```python
from build123d import *

# Parameters (mm, degrees)
SKETCH013_R     = 2.568486
PAD009_DEPTH    = 2.7
PAD009_FACE24_R = 2.568486
PAD010_DEPTH    = 6
SKETCH014_W     = 26.409815
SKETCH014_H     = 3.3
POCKET002_DEPTH = 17.5
FILLET004_R     = 15
FILLET005_R     = 4
FILLET006_R     = 6


with BuildPart() as part:
    # Sketch013 → Pad009 (new body)
    with BuildSketch(Plane.YZ.offset(2.7)):
        Polygon((20.516043, -0.037444), (30.366142, -1.649044), (35.213383, -1.649044), (36.83709, -1.959458), (38.007114, -2.29375), (38.389164, -2.413141), (39.177135, -2.866822), (39.72633, -3.224993), (40.275524, -3.63092), (40.967991, -4.299505), (41.254524, -4.729309), (41.923111, -5.636675), (41.923111, -12.869325), (41.062038, -14.015471), (40.035282, -14.922836), (39.032402, -15.710812), (37.838501, -16.236128), (36.525211, -16.133759), (35.140285, -16.133759), (6.593163, -16.133759), (-3.283293, -7.56256), (-3.283293, -0.110564), align=None)
        with Locations((35.551899, -9.23625)):
            Circle(SKETCH013_R, mode=Mode.SUBTRACT)
    extrude(amount=-PAD009_DEPTH)

    # Pad009 Face24 → Pad010 (add)
    with BuildSketch(Plane(origin=(2.7, 19.058053, -8.03373), x_dir=(0, -1, 0), z_dir=(1, 0, 0))):
        Polygon((-11.308089, -6.384686), (-1.45799, -7.996286), (22.341346, -7.923166), (22.341346, -0.47117), (12.46489, 8.100029), (-16.082232, 8.100029), (-17.467158, 8.100029), (-18.780448, 8.202398), (-19.974349, 7.677082), (-20.977229, 6.889106), (-22.003985, 5.981741), (-22.865058, 4.835595), (-22.865058, -2.397055), (-22.196471, -3.304421), (-21.909938, -3.734225), (-21.217471, -4.40281), (-20.668277, -4.808737), (-20.119082, -5.166908), (-19.331111, -5.620589), (-18.949061, -5.73998), (-17.779037, -6.074272), (-16.15533, -6.384686), align=None)
        with Locations((-16.493846, 1.20252)):
            Circle(PAD009_FACE24_R, mode=Mode.SUBTRACT)
    extrude(amount=PAD010_DEPTH)

    # Sketch014 (on Face46 of Pad010) → Pocket002 (cut, symmetric)
    with BuildSketch(Plane.YX.offset(16.133759)):
        with Locations((33.765693, 4.35)):
            Rectangle(SKETCH014_W, SKETCH014_H)
    extrude(amount=POCKET002_DEPTH, both=True, mode=Mode.SUBTRACT)

    # Fillet004
    fillet004_edges = [part.edges().sort_by_distance(p)[0] for p in [
        (5.7, 6.593163, -16.133759),
    ]]
    fillet(fillet004_edges, radius=FILLET004_R)

    # Fillet005
    fillet005_edges = [part.edges().sort_by_distance(p)[0] for p in [
        (4.35, 20.560785, -16.133759),
    ]]
    fillet(fillet005_edges, radius=FILLET005_R)

    # Fillet006
    fillet006_edges = [part.edges().sort_by_distance(p)[0] for p in [
        (5.7, -3.283293, -7.56256),
    ]]
    fillet(fillet006_edges, radius=FILLET006_R)


with BuildPart() as part_1:
    # Body005 placement: moved
    add(part.part.moved(Location((26.9, 0, 0))))


solid = part_1.part
```
For this review, take the finished solid that the model builds, in its own axes (mm). A direction names the side the tool comes from. Round coordinates to 2 decimals unless told otherwise and drop trailing zeros. Write each loop counter-clockwise with the first axis right and the second up, starting at its lowest first coordinate (ties: lowest second). Pieces come first, ordered by that corner, then holes. Notation, with made-up numbers: (61.25, 48) -> (68.25, 48) arc R12 ccw to (68.25, 69) -> close; hole circle Ø10 at (1.5, 59). An arc over 180 degrees is marked (long way). Use one line per item in the form item = value.
Q1. Consider section C-C (x = 31.75). State the section outline as (y, z) points.
Resolved:
outline = (-3.28, -4.83) arc R6 ccw to (-1.22, -9.36) -> (2.36, -12.46) arc R15 ccw to (12.19, -16.13) -> (16.56, -16.13) arc R4 ccw to (20.56, -12.13) -> (20.56, -0.04) -> (20.52, -0.04) -> (-3.28, -0.11) -> close
Q2. To check wall thickness, follow probe 1 along X at (y, z) = (24, -3.25); probe 2 along Y at (x, z) = (30.5, -4.75); probe 3 along Y at (x, z) = (28.25, -7). State the ranges of each line that lie inside material, in increasing order. Write a range as from..to.
Resolved:
probe_1 = 26.9..29.6, 32.9..35.6
probe_2 = -3.28..20.56
probe_3 = -2.88..34.29, 36.82..41.92
Q3. The part is to be moulded in two halves that separate along Y. For faces 6 (the cylindrical face through (31.311, 7.017, -15.212)), 7 (the flat face through (34.2, 36, -1.8)), 8 (the cylindrical face through (28.269, 36.737, -11.515)), say which applies: released by +Y, released by -Y, zero draft, split by the parting line, or undercut.
Resolved:
face_6 = released by -Y
face_7 = released by +Y
face_8 = undercut
Q4. Machinability: for faces 1 (the flat face through (31, -3.283, -2)), 2 (the flat face through (28, 33, -1.649)), 3 (the flat face through (28.231, 40.541, -14.476)), 4 (the flat face through (29, 24, -16.134)), 5 (the flat face through (31, 20.561, -6)), which of the approach directions +Z, -Z, +X, -X, +Y, -Y give a long, thin tool a straight path to every point of the face, cutting with its end or side? Answer none if there is none.
Resolved:
face_1 = +Z, -Z, +X, -X, -Y
face_2 = +Z, +X, -X, +Y
face_3 = -Z, +X, -X, +Y
face_4 = -Z, +X, -X, -Y
face_5 = +Z, -Z, +Y
Q5. Consider section D-D (x = 34.25). State the section outline as (y, z) points (1 decimal).
Resolved:
outline = (-3.3, -4.8) arc R6 ccw to (-1.2, -9.4) -> (2.4, -12.5) arc R15 ccw to (12.2, -16.1) -> (36.5, -16.1) -> (37.8, -16.2) -> (39, -15.7) -> (40, -14.9) -> (41.1, -14) -> (41.9, -12.9) -> (41.9, -5.6) -> (41.3, -4.7) -> (41, -4.3) -> (40.3, -3.6) -> (39.7, -3.2) -> (39.2, -2.9) -> (38.4, -2.4) -> (38, -2.3) -> (36.8, -2) -> (35.2, -1.6) -> (30.4, -1.6) -> (20.5, 0) -> (-3.3, -0.1) -> close; hole circle Ø5.1 at (35.6, -9.2)
Q6. Clearance check with flat-ended pins moving along their axes: pin 1 Ø1.4 at (x, y) = (35, 32.5) entering from +Z; pin 2 Ø3 at (y, z) = (35.55, -9.24) entering from -X; pin 3 Ø4 at (x, y) = (31.5, 32.5) entering from -Z. State where each tip first meets the part, or that it passes through.
Resolved:
pin_1 = -1.65
pin_2 = through
pin_3 = -16.13
Q7. Consider section B-B (z = -10). State the section outline as (x, y) points.
Resolved:
outline = (26.9, -0.47) -> (35.6, -0.47) -> (35.6, 33.1) -> (32.9, 33.1) -> (32.9, 20.56) -> (29.6, 20.56) -> (29.6, 33.1) -> (26.9, 33.1) -> close; (26.9, 38) -> (29.6, 38) -> (29.6, 41.92) -> (26.9, 41.92) -> close; (32.9, 38) -> (35.6, 38) -> (35.6, 41.92) -> (32.9, 41.92) -> close
Q8. Consider section A-A (y = 32). State the section outline as (x, z) points, then the cut area to 3 significant figures.
Resolved:
outline = (26.9, -16.13) -> (29.6, -16.13) -> (29.6, -1.65) -> (26.9, -1.65) -> close; (32.9, -16.13) -> (35.6, -16.13) -> (35.6, -1.65) -> (32.9, -1.65) -> close
area = 78.2 mm²
